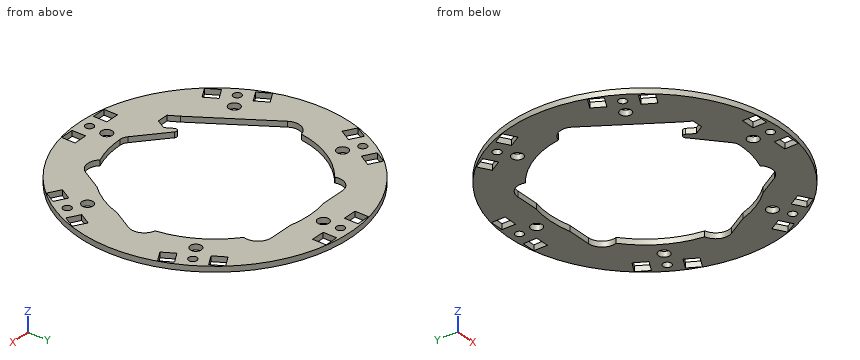
```python
from build123d import *

# Parameters (mm, degrees)
ESQUISSE1_R        = 50
ESQUISSE1_W        = 5
ESQUISSE1_H        = 5
ESQUISSE1_R_2      = 1.5
ESQUISSE1_R_3      = 2.05
BOSS_EXTRU_1_DEPTH = 2
SKETCH3_W          = 1
SKETCH3_H          = 8
CUT_EXTRUDE2_DEPTH = 10
CUT_EXTRUDE5_DEPTH = 10
FILLET1_R          = 1
FILLET2_R          = 4


with BuildPart() as part:
    # Esquisse1 → Boss.-Extru.1 (new body)
    with BuildSketch(Plane.XY):
        Circle(ESQUISSE1_R)
        Polygon((-39.762039705, -28.730127019), (-35.431912686, -26.230127019), (-32.931912686, -30.560254038), (-37.262039705, -33.060254038), align=None, mode=Mode.SUBTRACT)
        with Locations((-7.5, -46.3)):
            Rectangle(ESQUISSE1_W, ESQUISSE1_H, mode=Mode.SUBTRACT)
        with Locations((-40.096976195, -23.15)):
            Circle(ESQUISSE1_R_2, mode=Mode.SUBTRACT)
        Polygon((-42.931912686, -13.239745962), (-40.431912686, -17.569872981), (-44.762039705, -20.069872981), (-47.262039705, -15.739745962), align=None, mode=Mode.SUBTRACT)
        with Locations((-34.597845014, -19.975075133)):
            Circle(ESQUISSE1_R_3, mode=Mode.SUBTRACT)
        with BuildLine():
            ThreePointArc((-37.576499896, -2.739399901), (-35.858643923, 4.373966246), (-28.839360147, 2.304990085))
            Line((-28.839360147, 2.304990085), (-14.645940725, -25.367513459))
            Line((-14.645940725, -25.367513459), (-12.625214782, -28.867513459))
            Line((-12.625214782, -28.867513459), (-14.645940725, -32.367513459))
            Line((-14.645940725, -32.367513459), (-18.687392609, -32.367513459))
            Line((-18.687392609, -32.367513459), (-20.708118551, -28.867513459))
            Line((-20.708118551, -28.867513459), (-37.576499896, -2.739399901))
        make_face(mode=Mode.SUBTRACT)
        with Locations((-16.671397033, -9.625235564)):
            Circle(ESQUISSE1_R_3, mode=Mode.SUBTRACT)
        with Locations((0, -46.3)):
            Circle(ESQUISSE1_R_2, mode=Mode.SUBTRACT)
        with Locations((7.5, -46.3)):
            Rectangle(ESQUISSE1_W, ESQUISSE1_H, mode=Mode.SUBTRACT)
        with Locations((0, -39.950150265)):
            Circle(ESQUISSE1_R_3, mode=Mode.SUBTRACT)
        Polygon((32.931912686, -30.560254038), (35.431912686, -26.230127019), (39.762039705, -28.730127019), (37.262039705, -33.060254038), align=None, mode=Mode.SUBTRACT)
        with Locations((0, -19.232757636)):
            Circle(ESQUISSE1_R_3, mode=Mode.SUBTRACT)
        with Locations((16.666666667, -9.622504487)):
            Circle(ESQUISSE1_R_3, mode=Mode.SUBTRACT)
        with Locations((34.597845014, -19.975075132)):
            Circle(ESQUISSE1_R_3, mode=Mode.SUBTRACT)
        with BuildLine():
            ThreePointArc((20.996793686, -31.367513459), (14.166666667, -33.197640478), (12.336539648, -26.367513459))
            Line((12.336539648, -26.367513459), (29.003206314, 2.5))
            ThreePointArc((29.003206314, 2.5), (35.833333333, 4.330127019), (37.663460352, -2.5))
            Line((37.663460352, -2.5), (20.996793686, -31.367513459))
        make_face(mode=Mode.SUBTRACT)
        with Locations((40.096976195, -23.15)):
            Circle(ESQUISSE1_R_2, mode=Mode.SUBTRACT)
        Polygon((44.762039705, -20.069872981), (40.431912686, -17.569872981), (42.931912686, -13.239745962), (47.262039705, -15.739745962), align=None, mode=Mode.SUBTRACT)
        Polygon((-44.762039705, 20.069872981), (-40.431912686, 17.569872981), (-42.931912686, 13.239745962), (-47.262039705, 15.739745962), align=None, mode=Mode.SUBTRACT)
        with Locations((-40.096976195, 23.15)):
            Circle(ESQUISSE1_R_2, mode=Mode.SUBTRACT)
        with Locations((-34.597845014, 19.975075133)):
            Circle(ESQUISSE1_R_3, mode=Mode.SUBTRACT)
        with Locations((-16.671397032, 9.625235564)):
            Circle(ESQUISSE1_R_3, mode=Mode.SUBTRACT)
        Polygon((-32.931912686, 30.560254038), (-35.431912686, 26.230127019), (-39.762039705, 28.730127019), (-37.262039705, 33.060254038), align=None, mode=Mode.SUBTRACT)
        with Locations((0, 39.950150265)):
            Circle(ESQUISSE1_R_3, mode=Mode.SUBTRACT)
        with Locations((-7.5, 46.3)):
            Rectangle(ESQUISSE1_W, ESQUISSE1_H, mode=Mode.SUBTRACT)
        Circle(ESQUISSE1_R_3, mode=Mode.SUBTRACT)
        with Locations((16.669571796, 9.624181764)):
            Circle(ESQUISSE1_R_3, mode=Mode.SUBTRACT)
        with Locations((0, 19.165334425)):
            Circle(ESQUISSE1_R_3, mode=Mode.SUBTRACT)
        with Locations((34.597845014, 19.975075133)):
            Circle(ESQUISSE1_R_3, mode=Mode.SUBTRACT)
        Polygon((42.931912686, 13.239745962), (40.431912686, 17.569872981), (44.762039705, 20.069872981), (47.262039705, 15.739745962), align=None, mode=Mode.SUBTRACT)
        with Locations((40.096976195, 23.15)):
            Circle(ESQUISSE1_R_2, mode=Mode.SUBTRACT)
        with BuildLine():
            ThreePointArc((-16.666666667, 23.867513459), (-21.666666667, 28.867513459), (-16.666666667, 33.867513459))
            Line((-16.666666667, 33.867513459), (16.666666667, 33.867513459))
            ThreePointArc((16.666666667, 33.867513459), (21.666666667, 28.867513459), (16.666666667, 23.867513459))
            Line((16.666666667, 23.867513459), (-16.666666667, 23.867513459))
        make_face(mode=Mode.SUBTRACT)
        with Locations((0, 46.3)):
            Circle(ESQUISSE1_R_2, mode=Mode.SUBTRACT)
        with Locations((7.5, 46.3)):
            Rectangle(ESQUISSE1_W, ESQUISSE1_H, mode=Mode.SUBTRACT)
        Polygon((39.762039705, 28.730127019), (35.431912686, 26.230127019), (32.931912686, 30.560254038), (37.262039705, 33.060254038), align=None, mode=Mode.SUBTRACT)
    extrude(amount=BOSS_EXTRU_1_DEPTH)

    # Sketch3 → Cut-Extrude2 (cut)
    with BuildSketch(Plane.XY.offset(2)):
        with Locations((-10.5, 0)):
            Rectangle(SKETCH3_W, SKETCH3_H)
        with Locations((-22.833333333, 0)):
            Rectangle(SKETCH3_W, SKETCH3_H)
        Polygon((-13.233653965, 23.921361037), (-14.099679369, 23.421361037), (-12.349679369, 20.390272124), (-15.380768282, 18.640272124), (-14.880768282, 17.77424672), (-11.849679369, 19.52424672), (-10.099679369, 16.493157806), (-9.233653965, 16.993157806), (-10.983653965, 20.02424672), (-7.952565052, 21.77424672), (-8.452565052, 22.640272124), (-11.483653965, 20.890272124), align=None)
        Polygon((15.130768282, 18.207259422), (14.630768282, 17.341234018), (7.702565052, 21.341234018), (8.202565052, 22.207259422), align=None)
        Polygon((8.202565052, -22.207259422), (7.702565052, -21.341234018), (14.630768282, -17.341234018), (15.130768282, -18.207259422), align=None)
        Polygon((27.333333333, -0.5), (27.333333333, 0.5), (23.833333333, 0.5), (23.833333333, 4), (22.833333333, 4), (22.833333333, 0.5), (19.333333333, 0.5), (19.333333333, -0.5), (22.833333333, -0.5), (22.833333333, -4), (23.833333333, -4), (23.833333333, -0.5), align=None)
        Polygon((-14.099679369, -23.421361037), (-13.233653965, -23.921361037), (-11.483653965, -20.890272124), (-8.452565052, -22.640272124), (-7.952565052, -21.77424672), (-10.983653965, -20.02424672), (-9.233653965, -16.993157806), (-10.099679369, -16.493157806), (-11.849679369, -19.52424672), (-14.880768282, -17.77424672), (-15.380768282, -18.640272124), (-12.349679369, -20.390272124), align=None)
        Polygon((-20.834234776, 12.184801987), (-19.940304487, 11.668776346), (-20.102964744, 11.386925384), (-20.996895032, 11.902951025), (-21.517828526, 11.000607275), (-21.800380609, 11.163968654), (-21.279447115, 12.066312404), (-22.173377404, 12.582338045), (-22.010717147, 12.864189006), (-21.116786859, 12.348163365), (-20.596554487, 13.24840375), (-20.314002404, 13.085042371), align=None)
    extrude(amount=-CUT_EXTRUDE2_DEPTH, mode=Mode.SUBTRACT)

    # Sketch5 → Cut-Extrude5 (cut)
    with BuildSketch(Plane.XY.offset(2)):
        with BuildLine():
            Line((-16.642935498, -21.474029915), (-1.119551078, -34.759587589))
            ThreePointArc((-1.119551078, -34.759587589), (26.640402268, 22.355565101), (-34.426269912, 4.930949597))
            Line((-34.426269912, 4.930949597), (-16.642935498, -21.474029915))
        make_face()
    extrude(amount=-CUT_EXTRUDE5_DEPTH, mode=Mode.SUBTRACT)

    # Fillet1
    fillet1_edges = [part.edges().sort_by_distance(p)[0] for p in [
        (-16.642935498, -21.474029915, 1),
    ]]
    fillet(fillet1_edges, radius=FILLET1_R)

    # Fillet2
    fillet2_edges = [part.edges().sort_by_distance(p)[0] for p in [
        (-1.119551078, -34.759587589, 1),
    ]]
    fillet(fillet2_edges, radius=FILLET2_R)


solid = part.part
```
Design review of the part built by this model. Coordinates are the model's own, in mm. Give positions to 0.01 mm unless a question says otherwise; leave off trailing zeros. Write each loop counter-clockwise with the first axis right and the second up, starting at its lowest first coordinate (ties: lowest second). Pieces come first, ordered by that corner, then holes.
(1) Add section B-B (x = 30). Give the boundary of the cut face in (y, z), and give its area (3 significant figures).
Checked values:
outline: (-40, 0) - (-17.59, 0) - (-17.59, 2) - (-40, 2) - close; (17.59, 0) - (40, 0) - (40, 2) - (17.59, 2) - close
area: 89.6 mm2
(2) Add section A-A (y = 0). Give the boundary of the cut face in (x, z), and give its area (3 significant figures).
Checked values:
outline: (-50, 0) - (-38.38, 0) - (-38.38, 2) - (-50, 2) - close; (38.33, 0) - (50, 0) - (50, 2) - (38.33, 2) - close
area: 46.6 mm2
(3) Clearance check with flat-ended pins moving along their axes: pin 1 Ø0.6 at (x, z) = (-11.5, 1) entering from -Y; pin 2 Ø1 at (x, z) = (7, 1) entering from -Y; pin 3 Ø0.6 at (y, z) = (45, 1) entering from -X. State where each tip first meets the part, or that it passes through.
Checked values:
pin 1: stops at y = -48.73
pin 2: stops at y = -49.58
pin 3: stops at x = -22.4
(4) Wall thickness on line 1 along X through (y, z) = (19.5, 1.15) (3 decimals); line 2 along X through (y, z) = (-17, 1.6); line 3 along Y through (x, z) = (1, 0.25): over which ranges is each line inside the solid? List them lowest first.
Checked values:
line 1: x = -46.041 to -45.091, -43.775 to -36.592, -32.604 to -28.796, 28.796 to 32.604, 36.592 to 43.775, 45.091 to 46.041
line 2: x = -47.02 to -46.53, -40.76 to -28.37, 30.34 to 40.76, 46.53 to 47.02
line 3: y = -49.99 to -47.42, -45.18 to -41.74, -38.16 to -34.76, 34.76 to 38.16, 41.74 to 45.18, 47.42 to 49.99
(5) Add section D-D (z = 0.55). Give the number of separate pieces and of enclosed holes in the cut face, and give its area (3 significant figures).
Checked values:
separate pieces: 1
enclosed holes: 25
area: 3,540 mm2
(6) Add section C-C (y = -46.3). Give the boundary of the cut face in (x, z).
Checked values:
outline: (-18.88, 0) - (-10, 0) - (-10, 2) - (-18.88, 2) - close; (-5, 0) - (-1.5, 0) - (-1.5, 2) - (-5, 2) - close; (1.5, 0) - (5, 0) - (5, 2) - (1.5, 2) - close; (10, 0) - (18.88, 0) - (18.88, 2) - (10, 2) - close
